The listing builds one solid part. Answer for the finished solid, in the listing's coordinates (mm). Coordinates: 2 decimals unless noted, no trailing zeros. Write each loop counter-clockwise with the first axis right and the second up, starting at its lowest first coordinate (ties: lowest second). Pieces come first, ordered by that corner, then holes. Notation, with made-up numbers: M -13,9 L 38,9 A28 ccw 38,29 Z; hole C 34,81.5 d5. An arc over 180 degrees is marked long. Write item = value, one per line. Start each with the question number.
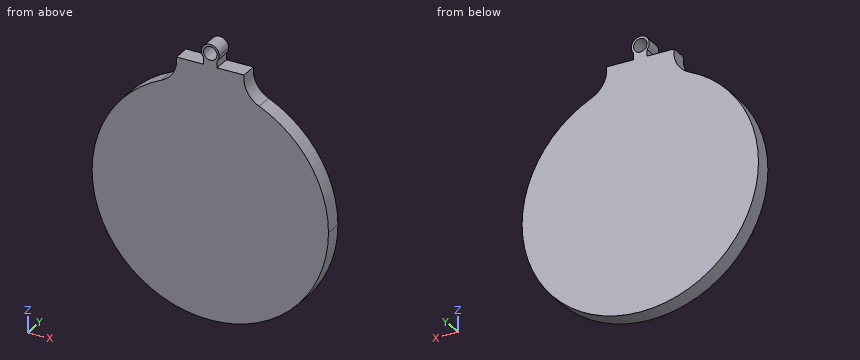
```python
from build123d import *

# Parameters (mm, degrees)
F0_R     = 2.54
F1_DEPTH = 6.35


with BuildPart() as f1:
    # F0 (on Front) → F1 (new body)
    with BuildSketch(Plane.XZ):
        with BuildLine():
            ThreePointArc((-18.35955, 40.481223), (-24.080288, -37.36231), (44.45, 0))
            ThreePointArc((44.45, 0), (37.36231, 24.080288), (18.35955, 40.481223))
            ThreePointArc((18.35955, 40.481223), (0, 44.45), (-18.35955, 40.481223))
        make_face()
        with BuildLine():
            ThreePointArc((-18.35955, 40.481223), (0, 44.45), (18.35955, 40.481223))
            ThreePointArc((18.35955, 40.481223), (13.86159, 44.619019), (12.7, 50.619328))
            Line((12.7, 50.619328), (2.54, 50.619328))
            Line((2.54, 50.619328), (0, 50.619328))
            Line((0, 50.619328), (-2.54, 50.619328))
            Line((-2.54, 50.619328), (-12.7, 50.619328))
            ThreePointArc((-12.7, 50.619328), (-13.86159, 44.619019), (-18.35955, 40.481223))
        make_face()
        with BuildLine():
            Line((0, 50.619328), (2.54, 50.619328))
            Line((2.54, 50.619328), (2.54, 53.159328))
            ThreePointArc((2.54, 53.159328), (0, 51.999384), (-2.54, 53.159328))
            Line((-2.54, 53.159328), (-2.54, 50.619328))
            Line((-2.54, 50.619328), (0, 50.619328))
        make_face()
        with BuildLine():
            ThreePointArc((-2.54, 53.159328), (0, 51.999384), (2.54, 53.159328))
            ThreePointArc((2.54, 53.159328), (3.149045, 54.185778), (3.360969, 55.360353))
            ThreePointArc((3.360969, 55.360353), (-1.174575, 58.509398), (-2.54, 53.159328))
        make_face()
        with Locations((0, 55.360353)):
            Circle(F0_R, mode=Mode.SUBTRACT)
    extrude(amount=F1_DEPTH)


solid = f1.part
```
1. The part is cut by section A-A, the plane x = 0. Write down the section's boundary in (y, z), and give its area (3 significant figures).
2. The part is cut by section D-D, the plane x = -22. Write down the section's boundary in (y, z).
3. The part is cut by section C-C, the plane z = 21.5. Write down the section's boundary in (x, y), and give its area (3 significant figures).
4. The part is cut by section B-B, the plane y = -2.5. Write down the section's boundary in (x, z), and give its area (3 significant figures).
5. Each of these flat-tipped pins is pushed along its axis until it touches: pin 1 (3 mm diameter, centred on x = 6, y = -3.5, fed in from +Z); pin 2 (3 mm diameter, centred on y = -4, z = 52.5, fed in from -X); pin 3 (2 mm diameter, centred on y = -4, z = 51.5, fed in from +X). Where does it stop, or does it pass through?
6. Straight lines are drawn through the part: L1, parallel to Z at x = 0, y = -2.5; L2, parallel to Z at x = -6.5, y = -2; L3, parallel to Z at x = 2, y = -0.25. For each, find the intervals that lie inside material, in ascending order. Write a range as [from, to].
Solution:
q1.outline = M -6.35,-44.45 L 0,-44.45 L 0,52.82 L -6.35,52.82 Z; M -6.35,57.9 L 0,57.9 L 0,58.72 L -6.35,58.72 Z
q1.area = 623 mm^2
q2.outline = M -6.35,-38.62 L 0,-38.62 L 0,38.62 L -6.35,38.62 Z
q3.outline = M -38.9,-6.35 L 38.9,-6.35 L 38.9,0 L -38.9,0 Z
q3.area = 494 mm^2
q4.outline = M -18.36,40.48 A44.45 ccw long 44.45,0 A44.45 ccw 18.36,40.48 A9.78 cw 12.7,50.62 L 2.54,50.62 L 2.54,53.16 A3.36 ccw 3.36,55.36 A3.36 ccw long -2.54,53.16 L -2.54,50.62 L -12.7,50.62 A9.78 cw Z; hole C 0,55.36 d5.08
q4.area = 6,420 mm^2
q5.pin_1 = 50.62
q5.pin_2 = -3.07
q5.pin_3 = 12.7
q6.L1 = [-44.45, 52.82], [57.9, 58.72]
q6.L2 = [-43.97, 50.62]
q6.L3 = [-44.4, 53.79], [56.93, 58.06]
